```python
from build123d import *

# Parameters (mm, degrees)
F0_W           = 48
F0_H           = 110
F1_DEPTH       = 7.5
F4_DEPTH       = 25
F6_D           = 5.5
F6_CBORE_D     = 8
F6_CBORE_DEPTH = 6


with BuildPart() as f1:
    # F0 (on Top) → F1 (new body, symmetric)
    with BuildSketch(Plane.XY):
        with Locations((9.722433, 22.829119)):
            Rectangle(F0_W, F0_H)
    extrude(amount=F1_DEPTH, both=True)

    # F3 (on face) → F4 (join)
    with BuildSketch(Plane.XY.offset(7.5)):
        with BuildLine():
            Line((-6.277567, 22.829119), (-6.277567, 77.829119))
            Line((-6.277567, 77.829119), (-14.277567, 77.829119))
            Line((-14.277567, 77.829119), (-14.277567, -32.170881))
            Line((-14.277567, -32.170881), (-14.071251, -32.170881))
            ThreePointArc((-14.071251, -32.170881), (-12.735921, -31.659805), (-12.083047, -30.387776))
            Line((-12.083047, -30.387776), (-6.277567, 22.829119))
        make_face()
        with BuildLine():
            Line((33.722433, 77.829119), (25.722433, 77.829119))
            Line((25.722433, 77.829119), (25.722433, 22.829119))
            Line((25.722433, 22.829119), (31.527912, -30.387776))
            ThreePointArc((31.527912, -30.387776), (32.180787, -31.659805), (33.516117, -32.170881))
            Line((33.516117, -32.170881), (33.722433, -32.170881))
            Line((33.722433, -32.170881), (33.722433, 77.829119))
        make_face()
    extrude(amount=F4_DEPTH)

    # F6 (through all)
    with Locations(Plane.XY.offset(7.5)):
        with Locations((9.722433, 42.829119), (9.722433, 62.829119), (9.722433, 2.829119), (9.722433, -17.170881)):
            CounterBoreHole(F6_D / 2, F6_CBORE_D / 2, F6_CBORE_DEPTH)


solid = f1.part
```
The listing builds one solid part. Answer for the finished solid, in the listing's coordinates (mm). A direction names the side the tool comes from. Coordinates: 2 decimals unless noted, no trailing zeros. Loops run counter-clockwise (first coordinate to the right, second up) from the corner with the lowest first, then second, coordinate; pieces in that order, holes last. Notation, with made-up numbers: (69, 63) - (115, 63) arc R9 ccw to (115, 76) - close; hole circle Ø8 at (58.25, 32.5). An arc over 180 degrees is marked (long way). Write item = value, one per line.
1) Section C-C (y = 33) is taken. Determine the outline of the cut face in (x, z).
Responses:
outline = (-14.28, -7.5) - (33.72, -7.5) - (33.72, 32.5) - (25.72, 32.5) - (25.72, 7.5) - (-6.28, 7.5) - (-6.28, 32.5) - (-14.28, 32.5) - close
2) Each of these flat-tipped pins is pushed along its axis until it touches: P1, Ø6.5, axis at x = 8, y = -16, coming from the +Z side; P2, Ø4, axis at x = 8.5, y = 2.5, coming from the +Z side. Where does it stop, or does it pass through?
Responses:
P1 = 7.5
P2 = 1.5
3) Which of the six approach directions +Z, -Z, +X, -X, +Y, -Y give full straight-line access (tool end or side, diameter ignored) to faces 4 (the face through (9, -20, 1.5)), 5 (the face through (-9.22, -4.15, 19.82)), 6 (the face through (-6.278, 50, 20))?
Responses:
face_4 = +Z
face_5 = +Z, -Y
face_6 = +Z, +Y, -Y
4) Section A-A (z = 30) is taken. Determine the outline of the cut face in (x, y), plus the area to 3 significant figures.
Responses:
outline = (-14.28, -32.17) - (-14.07, -32.17) arc R2 ccw to (-12.08, -30.39) - (-6.28, 22.83) - (-6.28, 77.83) - (-14.28, 77.83) - close; (25.72, 22.83) - (31.53, -30.39) arc R2 ccw to (33.52, -32.17) - (33.72, -32.17) - (33.72, 77.83) - (25.72, 77.83) - close
area = 1,430 mm^2
5) Section B-B (y = 4.5) is taken. Determine the outline of the cut face in (x, z).
Responses:
outline = (-14.28, -7.5) - (7.54, -7.5) - (7.54, 1.5) - (6.09, 1.5) - (6.09, 7.5) - (-8.28, 7.5) - (-8.28, 32.5) - (-14.28, 32.5) - close; (11.91, -7.5) - (33.72, -7.5) - (33.72, 32.5) - (27.72, 32.5) - (27.72, 7.5) - (13.36, 7.5) - (13.36, 1.5) - (11.91, 1.5) - close
6) Determine the mould class of faces 1 (the face through (11, -32.171, 1)), 2 (the face through (-10, 36, 32.5)), 3 (the face through (7.1, -16.34, -3.06)) for opening direction Y: pulls with the +Y half, pulls with the -Y half, needs draft (parallel to the pull), parting line crosses it, or undercut.
Responses:
face_1 = pulls with the -Y half
face_2 = needs draft
face_3 = undercut
7) Find the intervals of material crossed by line 1 along X through (y, z) = (68, 19); line 2 along Z through (x, y) = (0, -24); line 3 along X through (y, z) = (5.5, 10), in increasing order.
Responses:
line_1 = -14.28 to -6.28, 25.72 to 33.72
line_2 = -7.5 to 7.5
line_3 = -14.28 to -8.17, 27.61 to 33.72
8) Section D-D (z = -2) is taken. Determine the outline of the cut face in (x, y), plus the area to 3 significant figures.
Responses:
outline = (-14.28, -32.17) - (33.72, -32.17) - (33.72, 77.83) - (-14.28, 77.83) - close; hole circle Ø5.5 at (9.72, -17.17); hole circle Ø5.5 at (9.72, 2.83); hole circle Ø5.5 at (9.72, 42.83); hole circle Ø5.5 at (9.72, 62.83)
area = 5,180 mm^2
